Geometry: final body of the model. Coordinates: model frame, mm. Face numbers are marked on the shaded views. A direction names the side the tool comes from. Round coordinates to 2 decimals unless told otherwise and drop trailing zeros. Write each loop counter-clockwise with the first axis right and the second up, starting at its lowest first coordinate (ties: lowest second). Pieces come first, ordered by that corner, then holes. Notation, with made-up numbers: M -30.5,37.5 L -2.5,37.5 A6 ccw -2.5,46.5 Z; hole C -34.75,81 d9. An arc over 180 degrees is marked long. Use one line per item in the form item = value. Start each with the question number.
Item 1: Ray query, probe 1 along Z at (x, y) = (-3.5, -2); probe 2 along Z at (x, y) = (2.75, 7); probe 3 along X at (y, z) = (-7, 4). Return the intervals inside material, ascending.
Item 2: Section query D-D (y = -11). Return loops of the section in (x, z), and give its area (3 significant figures).
Item 3: Section query B-B (z = 0). Return loops of the section in (x, y), and give its area (3 significant figures).
Item 4: Pin query (flat end, axial travel): pin 1 Ø4 at (x, z) = (-1, -3.5) entering from +Y; pin 2 Ø1.5 at (x, y) = (-3, 22.5) entering from -Z; pin 3 Ø3 at (y, z) = (21.5, -3.5) entering from -X. Return the tip coordinate at first contact, or that it passes through.
Item 5: Section query C-C (y = 9). Return loops of the section in (x, z).
Item 6: Reachability of the marked faces 1 and 2 from +Z, -Z, +X, -X, +Y, -Y: full face, straight path, thin tool, end or side. Return the list, or none.
Item 7: Section query A-A (x = 0). Return loops of the section in (y, z).
from build123d import *

# Parameters (mm, degrees)
SKETCH1_R      = 3.8
EXTRUDE1_DEPTH = 25
SKETCH2_R      = 4.75
EXTRUDE2_DEPTH = 20.25


with BuildPart() as part:
    # Sketch1 → Extrude1 (new body)
    with BuildSketch(Plane(origin=(0, 0, 0), x_dir=(1, 0, 0), z_dir=(0, 1, 0))):
        Circle(SKETCH1_R)
    extrude(amount=EXTRUDE1_DEPTH)

    # Sketch2 → Extrude2 (add)
    with BuildSketch(Plane.XZ):
        Circle(SKETCH2_R)
    extrude(amount=EXTRUDE2_DEPTH)

    # Sketch3 → Revolve1 (revolve)
    with BuildSketch(Plane(origin=(0, 0, 0), x_dir=(0, 0, -1), z_dir=(1, 0, 0))):
        with BuildLine():
            Line((0, -25), (0, -20.25))
            Line((0, -20.25), (-4.75, -20.25))
            ThreePointArc((-4.75, -20.25), (-3.358757211, -23.608757211), (0, -25))
        make_face()
    revolve(axis=Axis((0, -25.519108832, 0), (0, 1, 0)))

    # Sketch4 → Revolve2 (revolve)
    with BuildSketch(Plane(origin=(0, 0, 0), x_dir=(0, 0, -1), z_dir=(1, 0, 0))):
        Polygon((0, 25), (3.8, 25), (1.9, 38), (0, 38), align=None)
    revolve(axis=Axis((0, 39.39190429, 0), (0, -1, 0)))


solid = part.part
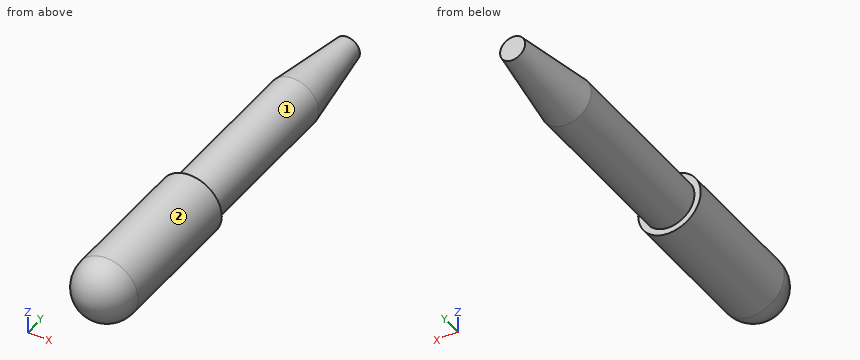
Working result:
q1.probe_1 = -3.21 to 3.21
q1.probe_2 = -2.62 to 2.62
q1.probe_3 = -2.56 to 2.56
q2.outline = C 0,0 d9.5
q2.area = 70.9 mm²
q3.outline = M -4.75,-20.25 A4.75 ccw 4.75,-20.25 L 4.75,0 L 3.8,0 L 3.8,25 L 1.9,38 L -1.9,38 L -3.8,25 L -3.8,0 L -4.75,0 Z
q3.area = 492 mm²
q4.pin_1 = 38
q4.pin_2 = -3.06
q4.pin_3 = -3.23
q5.outline = C 0,0 d7.6
q6.face_1 = +Y
q6.face_2 = +Y, -Y
q7.outline = M -20.25,-4.75 L 0,-4.75 L 0,-3.8 L 25,-3.8 L 38,-1.9 L 38,1.9 L 25,3.8 L 0,3.8 L 0,4.75 L -20.25,4.75 A4.75 ccw Z
